The drawing under review shows one solid part. Ordinate dimensions are in mm from its lowest x, y, z. A direction names the side the tool comes from. Coordinates: 2 decimals unless noted, no trailing zeros. Write each loop counter-clockwise with the first axis right and the second up, starting at its lowest first coordinate (ties: lowest second). Pieces come first, ordered by that corner, then holes. Notation, with made-up numbers: (-13, -22) -> (41, -22) arc R32 ccw to (41, 17) -> close; hole circle Ø7 at (-0.75, 44.25). An arc over 180 degrees is marked (long way). One line per question, with ' | ' between items. Start each with the question number.
Q1. Add section A-A on y = 15.75. State the section outline as (x, z) points.
Q2. Wall thickness on probe 1 along X at (y, z) = (6.5, 11.75); probe 2 along Z at (x, y) = (17.5, 28); probe 3 along Y at (x, z) = (27, 2.25): over which ranges is each line inside the solid? List them lowest first.
Q3. For P1, Ø6, axis at y = 19.5, z = 5, coming from the +X side; P2, Ø5, axis at x = 42.5, y = 13.5, coming from the -Z side; P3, Ø5.5, axis at y = 8.5, z = 14, coming from the -X side, all flat-tipped, find the tip position at first contact; note any pin that passes through.
Q4. Draft analysis for pull direction X (two halves, no side actions). For the marked faces 1, 2 and 3, state which applies: pulls with the +X half, pulls with the -X half, needs draft (parallel to the pull), parting line crosses it, or undercut.
Q5. For the marked faces 4, 5, 6 and 7, list the 3-axis set-ups (+Z, -Z, +X, -X, +Y, -Y) from which the entire face can be reached by the end or side of a thin tool; tool diameter is ignored.
Q6. Add section D-D on x = 5. State the section outline as (y, z) points.
Q7. Add section B-B on x = 12. State the section outline as (y, z) points.
Q8. Add section C-C on z = 16.75. State the section outline as (x, y) points, and give its area (3 significant figures).
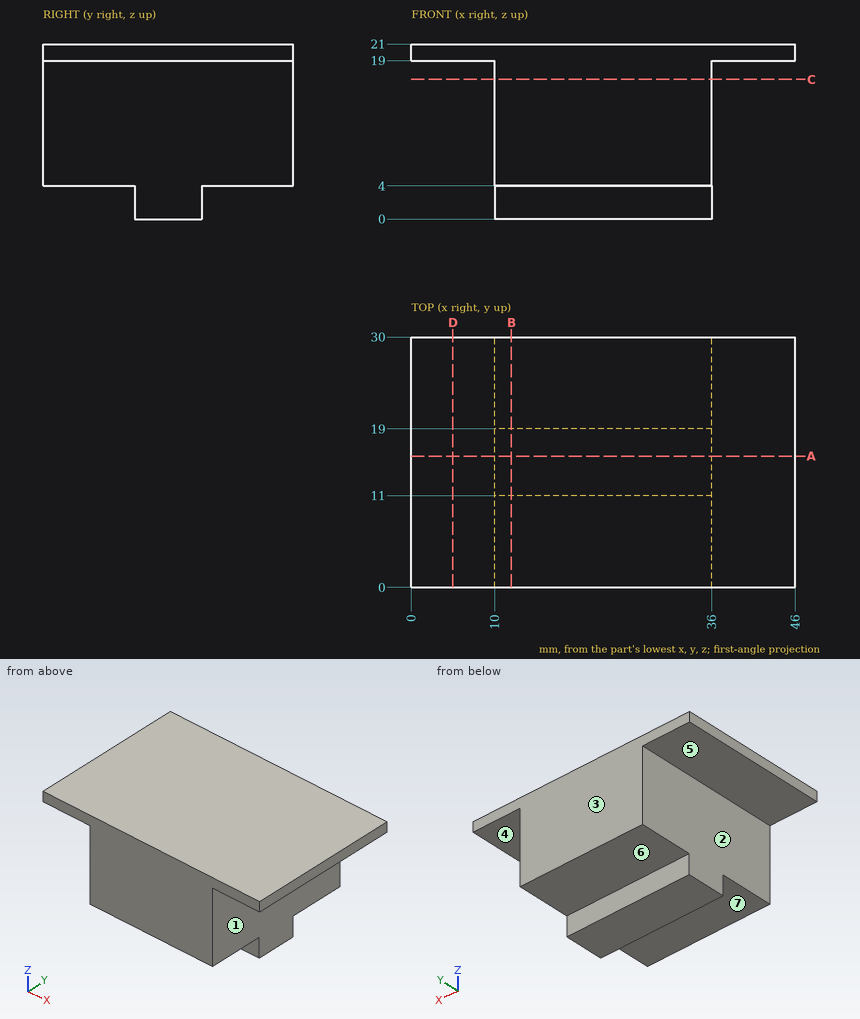
Output values:
1) outline: (0, 19) -> (10, 19) -> (10, 0) -> (36, 0) -> (36, 19) -> (46, 19) -> (46, 21) -> (0, 21) -> close
2) probe 1: x = 10 to 36 | probe 2: z = 4 to 21 | probe 3: y = 11 to 19
3) P1: stops at x = 36 | P2: stops at z = 19 | P3: stops at x = 10
4) face 1: pulls with the +X half | face 2: pulls with the -X half | face 3: needs draft
5) face 4: -Z, +X, +Y, -Y | face 5: -Z, -X, +Y, -Y | face 6: -Z, +X, -X, +Y | face 7: -Z, +X, -X, -Y
6) outline: (0, 19) -> (30, 19) -> (30, 21) -> (0, 21) -> close
7) outline: (0, 4) -> (11, 4) -> (11, 0) -> (19, 0) -> (19, 4) -> (30, 4) -> (30, 21) -> (0, 21) -> close
8) outline: (10, 0) -> (36, 0) -> (36, 30) -> (10, 30) -> close | area: 780 mm2
